from build123d import *

# Parameters (mm, degrees)
SKETCH_R        = 25
PAD_DEPTH       = 25
PAD_TAPER       = 15
SKETCH001_R     = 20.195
POCKET_DEPTH    = 20
POCKET_TAPER    = 15
SKETCH002_R     = 10
PAD001_DEPTH    = 20
PAD001_TAPER    = 18
SKETCH003_R     = 1.75
POCKET001_DEPTH = 17


with BuildPart() as part:
    # Sketch → Pad (new body)
    with BuildSketch(Plane.XY):
        Circle(SKETCH_R)
    extrude(amount=PAD_DEPTH, taper=PAD_TAPER)

    # Sketch001 (on Face2 of Pad) → Pocket (cut)
    with BuildSketch(Plane(origin=(0, 0, 0), x_dir=(1, 0, 0), z_dir=(0, 0, -1))):
        Circle(SKETCH001_R)
    extrude(amount=-POCKET_DEPTH, taper=POCKET_TAPER, mode=Mode.SUBTRACT)

    # Sketch002 (on Face5 of Pocket) → Pad001 (join)
    with BuildSketch(Plane(origin=(0, 0, 20), x_dir=(1, 0, 0), z_dir=(0, 0, -1))):
        Circle(SKETCH002_R)
    extrude(amount=PAD001_DEPTH, taper=PAD001_TAPER)

    # Sketch003 (on Face7 of Pad001) → Pocket001 (cut)
    with BuildSketch(Plane(origin=(0, 0, 0), x_dir=(1, 0, 0), z_dir=(0, 0, -1))):
        Circle(SKETCH003_R)
    extrude(amount=-POCKET001_DEPTH, mode=Mode.SUBTRACT)


solid = part.part
Could you check a few things on this model? Use its own coordinates, in mm. A direction names the side the tool comes from. Give positions to 0.01 mm unless a question says otherwise; leave off trailing zeros. Order: outer loops, then holes, each group sorted by start corner. A loop starts at its lowest first (then second) coordinate and runs counter-clockwise, first axis right, second up.
Item 1: If we section it at C-C, the plane z = 16: Write out the boundary of the cut face in (x, y).
Item 2: If we section it at A-A, the plane x = 0: Write out the boundary of the cut face in (y, z) (3 decimals), plus the area to 3 significant figures.
Item 3: If we mould it in two halves opening along Y, with no side actions, what happens to faces 3 (the face through (9.282, -17.846, 18.231)), 4 (the face through (-16.271, -0.716, 14.584)), 5 (the face through (0, 0, 25))? For each: pulls with the +Y half, pulls with the -Y half, needs draft (parallel to the pull), parting line crosses it, or undercut.
Item 4: I'm going to push flat-ended pins straight in: pin 1 (1 mm diameter, centred on y = -11.5, z = 21.5, fed in from -X); pin 2 (1.5 mm diameter, centred on x = 7, y = -10, fed in from -Z); pin 3 (12 mm diameter, centred on y = -12, z = 21.5, fed in from -X). Where does each tip first touch, or does it pass through?
Item 5: For faces 1 (the face through (1.617, 0.67, 8.381)), 2 (the face through (-2, -20.3, 0)), which set-ups out of +Z, -Z, +X, -X, +Y, -Y let a thin tool reach every point of the face, with its end or its side?
Item 6: I need wall thicknesses on line 1 (Y direction, x = 0, z = 9); line 2 (Y direction, x = 0, z = 9.5); line 3 (Y direction, x = 3, z = 7). Which ranges of each line are inside material? Lowest first, please.
Item 7: If we section it at B-B, the plane z = 10: Write out the boundary of the cut face in (x, y), plus the area to 3 significant figures.
Values:
1. outline: circle Ø41.43 at (0, 0); circle Ø17.4 at (0, 0); hole circle Ø31.82 at (0, 0); hole circle Ø3.5 at (0, 0)
2. outline: (-25, 0) - (-20.195, 0) - (-14.836, 20) - (-10, 20) - (-3.502, 0) - (-1.75, 0) - (-1.75, 17) - (1.75, 17) - (1.75, 0) - (3.502, 0) - (10, 20) - (14.836, 20) - (20.195, 0) - (25, 0) - (18.301, 25) - (-18.301, 25) - close
2. area: 592 mm2
3. face 3: parting line crosses it
3. face 4: undercut
3. face 5: needs draft
4. pin 1: stops at x = -15.82
4. pin 2: stops at z = 20
4. pin 3: stops at x = -18.88
5. face 1: -Z
5. face 2: -Z, +X, -X, +Y, -Y
6. line 1: y = -22.59 to -17.78, -6.43 to -1.75, 1.75 to 6.43, 17.78 to 22.59
6. line 2: y = -22.45 to -17.65, -6.59 to -1.75, 1.75 to 6.59, 17.65 to 22.45
6. line 3: y = -22.93 to -18.07, -4.94 to 4.94, 18.07 to 22.93
7. outline: circle Ø44.64 at (0, 0); circle Ø13.5 at (0, 0); hole circle Ø35.03 at (0, 0); hole circle Ø3.5 at (0, 0)
7. area: 735 mm2
